from build123d import *

# Parameters (mm, degrees)
F0_W      = 25
F0_H      = 11
F1_DEPTH  = 10
F2_R      = 8
F3_DEPTH  = 3
F4_R      = 6
F5_DEPTH  = 9
F6_W      = 11
F6_H      = 10
F7_DEPTH  = 2
F8_W      = 11
F8_H      = 10
F9_DEPTH  = 2
F10_R     = 5
F11_R     = 1.75
F12_DEPTH = 25
F13_R     = 8.25
F14_DEPTH = 3


with BuildPart() as f1:
    # F0 (on Top) → F1 (new body)
    with BuildSketch(Plane.XY):
        with Locations((12.5, 5.5)):
            Rectangle(F0_W, F0_H)
    extrude(amount=F1_DEPTH)

    # F2 (on face) → F3 (cut)
    with BuildSketch(Plane.XZ):
        with Locations((12.5, 10)):
            Circle(F2_R)
    extrude(amount=-F3_DEPTH, mode=Mode.SUBTRACT)

    # F4 (on face) → F5 (cut)
    with BuildSketch(Plane(origin=(0, 11, 0), x_dir=(-1, 0, 0), z_dir=(0, 1, 0))):
        with Locations((-12.5, 10)):
            Circle(F4_R)
    extrude(amount=-F5_DEPTH, mode=Mode.SUBTRACT)

    # F6 (on face) → F7 (join)
    with BuildSketch(Plane(origin=(0, 0, 0), x_dir=(0, -1, 0), z_dir=(-1, 0, 0))):
        with Locations((-5.5, 5)):
            Rectangle(F6_W, F6_H)
    extrude(amount=F7_DEPTH)

    # F8 (on face) → F9 (join)
    with BuildSketch(Plane.YZ.offset(25)):
        with Locations((5.5, 5)):
            Rectangle(F8_W, F8_H)
    extrude(amount=F9_DEPTH)

    # F10
    f10_edges = [f1.edges().sort_by_distance(p)[0] for p in [
        (27, 11, 5),
        (27, 0, 5),
        (-2, 11, 5),
        (-2, 0, 5),
    ]]
    fillet(f10_edges, radius=F10_R)

    # F11 (on face) → F12 (cut)
    with BuildSketch(Plane.XY.offset(10)):
        with Locations((0.75, 6.25)):
            Circle(F11_R)
        with Locations((24.25, 6.25)):
            Circle(F11_R)
    extrude(amount=-F12_DEPTH, mode=Mode.SUBTRACT)

    # F13 (on face) → F14 (cut)
    with BuildSketch(Plane(origin=(0, 11, 0), x_dir=(-1, 0, 0), z_dir=(0, 1, 0))):
        with Locations((-12.5, 10)):
            Circle(F13_R)
    extrude(amount=-F14_DEPTH, mode=Mode.SUBTRACT)


solid = f1.part
Design review of the part built by this model. Coordinates are the model's own, in mm. A direction names the side the tool comes from. Round coordinates to 2 decimals unless told otherwise and drop trailing zeros. Write each loop counter-clockwise with the first axis right and the second up, starting at its lowest first coordinate (ties: lowest second). Pieces come first, ordered by that corner, then holes. Notation, with made-up numbers: (-31.5, 48) -> (-26.5, 48) arc R29 cw to (-26.5, 71) -> close; hole circle Ø4 at (-29, -18.5). An arc over 180 degrees is marked (long way). One line per item, written item: value. Start each with the question number.
Q1. Add section C-C (y = 7). Give the boundary of the cut face in (x, z).
Q2. Tool access review of faces 4 (the face through (12.324, 1.479, 2.002)), 5 (the face through (25, 1, 5)), 6 (the face through (14, 8, 4)): name each direction out of +Z, -Z, +X, -X, +Y, -Y from which nothing blocks a thin tool from reaching the whole face with its end or side.
Q3. Insertion check: P1, Ø3, axis at x = 24.25, y = 6.25, coming from the -Z side; P2, Ø4, axis at x = 1, y = 7, coming from the -Z side; P3, Ø4, axis at x = 13, z = 4.5, coming from the +Y side. Each pin has a flat end and moves straight along its axis. Give the tip position at first contact, or say it passes through.
Q4. Add section B-B (z = 4.75). Give the boundary of the cut face in (x, y).
Q5. The part is to be moulded in two halves that separate along Y. For faces 1 (the face through (22.86, 5.19, 5.07)), 2 (the face through (12, 5, 0)), 3 (the face through (11, 3, 4)), say which applies: pulls with the +Y half, pulls with the -Y half, needs draft (parallel to the pull), parting line crosses it, or undercut.
Q6. Add section D-D (x = 0.75). Give the boundary of the cut face in (y, z).
Q7. Add section A-A (x = 12.5). Give the boundary of the cut face in (y, z).
Q8. To check wall thickness, follow probe 1 along X at (y, z) = (5, 3.5); probe 2 along X at (y, z) = (5, 7.5); probe 3 along X at (y, z) = (2, 7). State the ranges of each line that lie inside material, in increasing order.
Response:
1. outline: (-1.9, 0) -> (-0.83, 0) -> (-0.83, 10) -> (-1.9, 10) -> close; (2.33, 0) -> (22.67, 0) -> (22.67, 10) -> (18.5, 10) arc R6 cw to (6.5, 10) -> (2.33, 10) -> close; (25.83, 0) -> (26.9, 0) -> (26.9, 10) -> (25.83, 10) -> close
2. face 4: +Z, -Y
2. face 5: +Z, -Z, +X, -Y
2. face 6: +Z, +Y
3. P1: passes through
3. P2: stops at z = 0
3. P3: stops at y = 8
4. outline: (-2, 5) arc R5 ccw to (3, 0) -> (6.46, 0) -> (6.46, 3) -> (9.6, 3) -> (9.6, 8) -> (6.14, 8) -> (6.14, 11) -> (3, 11) arc R5 ccw to (-2, 6) -> close; (15.4, 3) -> (18.54, 3) -> (18.54, 0) -> (22, 0) arc R5 ccw to (27, 5) -> (27, 6) arc R5 ccw to (22, 11) -> (18.86, 11) -> (18.86, 8) -> (15.4, 8) -> close; hole circle Ø3.5 at (0.75, 6.25); hole circle Ø3.5 at (24.25, 6.25)
5. face 1: undercut
5. face 2: needs draft
5. face 3: pulls with the -Y half
6. outline: (0.53, 0) -> (4.5, 0) -> (4.5, 10) -> (0.53, 10) -> close; (8, 0) -> (10.47, 0) -> (10.47, 10) -> (8, 10) -> close
7. outline: (0, 0) -> (11, 0) -> (11, 1.75) -> (8, 1.75) -> (8, 4) -> (3, 4) -> (3, 2) -> (0, 2) -> close
8. probe 1: x = -2 to -0.47, 1.97 to 23.03, 25.47 to 27
8. probe 2: x = -2 to -0.47, 1.97 to 7.05, 17.95 to 23.03, 25.47 to 27
8. probe 3: x = -1 to 5.08, 19.92 to 26
